Geometry: final body of the model. Coordinates: model frame, mm. A direction names the side the tool comes from. Give positions to 0.01 mm unless a question says otherwise; leave off trailing zeros. Loops run counter-clockwise (first coordinate to the right, second up) from the corner with the lowest first, then second, coordinate; pieces in that order, holes last. Notation, with made-up numbers: M -14.5,89 L -3.5,89 A18 cw -3.5,104 Z; hole C 59.5,52.5 d10. An arc over 180 degrees is marked long. Put each result on its own line as item: value.
```python
from build123d import *

# Parameters (mm, degrees)
F0_W     = 478
F0_H     = 388
F1_DEPTH = 110
F2_W     = 400
F2_H     = 19
F3_DEPTH = 502
F4_W     = 400
F4_H     = 6
F5_DEPTH = 502
F7_DEPTH = 559


with BuildPart() as f1:
    # F0 (on Top) → F1 (new body)
    with BuildSketch(Plane.XY):
        Polygon((0, 0), (0, 400), (-502, 400), (-502, 0), (-521, 0), (-521, -19), (9, -19), (9, 0), align=None)
        with Locations((-251, 194)):
            Rectangle(F0_W, F0_H, mode=Mode.SUBTRACT)
    extrude(amount=-F1_DEPTH)

    # F2 (on Right) → F3 (cut)
    with BuildSketch(Plane.YZ):
        with Locations((200, -100.5)):
            Rectangle(F2_W, F2_H)
        with Locations((200, -9.5)):
            Rectangle(F2_W, F2_H)
    extrude(amount=-F3_DEPTH, mode=Mode.SUBTRACT)

    # F4 (on Right) → F5 (join)
    with BuildSketch(Plane.YZ):
        with Locations((200, -81.88692)):
            Rectangle(F4_W, F4_H)
    extrude(amount=-F5_DEPTH)

    # F6 (on Right) → F7 (cut, symmetric)
    with BuildSketch(Plane.YZ):
        Polygon((-10, -110), (0, -110), (0, -100), align=None)
    extrude(amount=F7_DEPTH, both=True, mode=Mode.SUBTRACT)


solid = f1.part
```
Item 1: Section C-C on z = -68. Output: boundary loops of the cut face in (x, y), then the cut area to 3 significant figures.
Output values:
outline: M -521,-19 L 9,-19 L 9,0 L 0,0 L 0,400 L -502,400 L -502,0 L -521,0 Z; hole M -490,0 L -12,0 L -12,388 L -490,388 Z
area: 25,400 mm²
Item 2: Section A-A on x = -365. Output: boundary loops of the cut face in (y, z), then the cut area to 3 significant figures.
Output values:
outline: M -19,-110 L -10,-110 L 0,-100 L 0,-84.89 L 388,-84.89 L 388,-91 L 400,-91 L 400,-19 L 388,-19 L 388,-78.89 L 0,-78.89 L 0,0 L -19,0 Z
area: 5,230 mm²
Item 3: Set-up query: faces 4 (the flat face through (-252, 0, -49)), 5 (the flat face through (-248, 191, -84.887)), 6 (the flat face through (-248, 191, -78.887)). Return all of +Z, -Z, +X, -X, +Y, -Y with unobstructed straight access to the full face (end or side cutting, diameter ignored); none if empty.
Output values:
face 4: none
face 5: -Z
face 6: +Z
Item 4: Mould query, pull axis Y, two halves, no side actions, for faces 1 (the flat face through (-12, 191, -49)), 2 (the flat face through (-502, 203, -54)), 3 (the flat face through (-260, -19, -54)). Classes: pulls with the +Y half, pulls with the -Y half, needs draft (parallel to the pull), parting line crosses it, or undercut.
Output values:
face 1: undercut
face 2: needs draft
face 3: pulls with the -Y half
Item 5: Line query: probe 1 along X at (y, z) = (102.5, -85); probe 2 along Y at (x, z) = (-156.5, -66); probe 3 along Z at (x, y) = (-203.5, 145.5). Output: solid intervals per line, ascending. Write a range as [from, to].
Output values:
probe 1: [-502, -490], [-12, 0]
probe 2: [-19, 0], [388, 400]
probe 3: [-84.89, -78.89]
Item 6: Pin query (flat end, axial travel): pin 1 Ø5 at (y, z) = (105.5, -16) entering from -X; pin 2 Ø8 at (x, y) = (-208.5, 168) entering from +Z; pin 3 Ø6 at (y, z) = (235, -81) entering from -X; pin 4 Ø6 at (x, y) = (-53.5, 350) entering from -Z. Return the tip coordinate at first contact, or that it passes through.
Output values:
pin 1: through
pin 2: z = -78.89
pin 3: x = -502
pin 4: z = -84.89
Item 7: Section B-B on y = 36.5. Output: boundary loops of the cut face in (x, z), then the cut area to 3 significant figures.
Output values:
outline: M -502,-91 L -490,-91 L -490,-84.89 L -12,-84.89 L -12,-91 L 0,-91 L 0,-19 L -12,-19 L -12,-78.89 L -490,-78.89 L -490,-19 L -502,-19 Z
area: 4,600 mm²
